```python
from build123d import *

# Parameters (mm, degrees)
SKETCH_11_W         = 15
SKETCH_11_H         = 15
SKETCH_11_W_2       = 13
SKETCH_11_H_2       = 13
F_15X15X1_1_DEPTH   = 100
SKETCH_12_R         = 1.45
CUT_EXTRUDE_1_DEPTH = 22
SKETCH_13_R         = 4
SKETCH_13_R_2       = 1.45
CUT_EXTRUDE_2_DEPTH = 102.396498953


with BuildPart() as part:
    # 草图11 → 铝管 15X15X1(1) (new body)
    with BuildSketch(Plane.YZ):
        Rectangle(SKETCH_11_W, SKETCH_11_H)
        Rectangle(SKETCH_11_W_2, SKETCH_11_H_2, mode=Mode.SUBTRACT)
    extrude(amount=F_15X15X1_1_DEPTH)

    # 草图12 → 切除-拉伸1 (cut)
    with BuildSketch(Plane.XY.offset(7.5)):
        with Locations((33, 0)):
            Circle(SKETCH_12_R)
    extrude(amount=-CUT_EXTRUDE_1_DEPTH, mode=Mode.SUBTRACT)

    # 草图13 → 切除-拉伸2 (cut, through all)
    with BuildSketch(Plane.XY.offset(7.5)):
        with Locations((90, 0)):
            Circle(SKETCH_13_R)
        with Locations((80, 0)):
            Circle(SKETCH_13_R_2)
        with Locations((70, 0)):
            Circle(SKETCH_13_R_2)
    extrude(amount=-CUT_EXTRUDE_2_DEPTH, mode=Mode.SUBTRACT)


solid = part.part
```
The listing builds one solid part. Answer for the finished solid, in the listing's coordinates (mm). A direction names the side the tool comes from. Coordinates: 2 decimals unless noted, no trailing zeros. Loops run counter-clockwise (first coordinate to the right, second up) from the corner with the lowest first, then second, coordinate; pieces in that order, holes last. Notation, with made-up numbers: (47.5, -0.75) -> (77.5, -0.75) arc R17 ccw to (77.5, 17.25) -> close; hole circle Ø2 at (6, 15.25). An arc over 180 degrees is marked (long way). Use one line per item in the form item = value. Start each with the question number.
Item 1: Consider L1, parallel to Y at x = 34, z = 2.25; L2, parallel to Y at x = 33, z = 6.85. Determine where each line is inside the solid, lowest interval first. Write a range as [from, to].
Item 2: The part is cut by section C-C on y = -2.5. Determine the outline of the cut face in (x, z).
Item 3: The part is cut by section A-A on x = 29. Determine the outline of the cut face in (y, z).
Item 4: The part is cut by section B-B on z = -2.75. Determine the outline of the cut face in (x, y), then the cut area to 3 significant figures.
Item 5: A tool of negligible diameter and unlimited length cuts with its end or side. For faces 4 (the face through (49, -6.5, 0)), 5 (the face through (68.85, -0.88, 7.01)), from which of +Z, -Z, +X, -X, +Y, -Y can it reach the whole face along a straight path? Write none if from no direction.
Item 6: The mould has two halves that part along Y. Classify faces 1 (the face through (49, 7.5, 0)), 2 (the face through (86, 0, -7)), 3 (the face through (49, 0, -7.5)): released by +Y, released by -Y, zero draft, split by the parting line, or undercut.
Answer key:
q1.L1 = [-7.5, -6.5], [6.5, 7.5]
q1.L2 = [-7.5, -1.45], [1.45, 7.5]
q2.outline = (0, -7.5) -> (86.88, -7.5) -> (86.88, -6.5) -> (0, -6.5) -> close; (0, 6.5) -> (86.88, 6.5) -> (86.88, 7.5) -> (0, 7.5) -> close; (93.12, -7.5) -> (100, -7.5) -> (100, -6.5) -> (93.12, -6.5) -> close; (93.12, 6.5) -> (100, 6.5) -> (100, 7.5) -> (93.12, 7.5) -> close
q3.outline = (-7.5, -7.5) -> (7.5, -7.5) -> (7.5, 7.5) -> (-7.5, 7.5) -> close; hole (-6.5, -6.5) -> (6.5, -6.5) -> (6.5, 6.5) -> (-6.5, 6.5) -> close
q4.outline = (0, -7.5) -> (100, -7.5) -> (100, -6.5) -> (0, -6.5) -> close; (0, 6.5) -> (100, 6.5) -> (100, 7.5) -> (0, 7.5) -> close
q4.area = 200 mm2
q5.face_4 = +X, -X
q5.face_5 = +Z, -Z
q6.face_1 = released by +Y
q6.face_2 = undercut
q6.face_3 = zero draft
